Source: CAD feature listing. Evaluate the final solid. Frame: model axes, mm. Face numbers are marked on the shaded views. A direction names the side the tool comes from. Round coordinates to 2 decimals unless told otherwise and drop trailing zeros. Order: outer loops, then holes, each group sorted by start corner. A loop starts at its lowest first (then second) coordinate and runs counter-clockwise, first axis right, second up. Notation, with made-up numbers: (-26.5, 33.25) - (15.5, 33.25) arc R17 cw to (15.5, 37.25) - close; hole circle Ø8 at (-5, 14.5). An arc over 180 degrees is marked (long way). Put each result on its own line as item: value. Start each with the question number.
1) Access query for the marked faces 4 and 5. Directions: +Z, -Z, +X, -X, +Y, -Y. A direction counts if a zero-diameter tool reaches every point of the face in a straight line with its end or side. Return the directions, or none.
2) Section A-A on x = 5. Output: boundary loops of the cut face in (y, z).
3) Line query: probe 1 along X at (y, z) = (-2.5, 4); probe 2 along Z at (x, y) = (5, -8); probe 3 along X at (y, z) = (10.75, 5.25). Output: solid intervals per line, ascending. Write a range as [from, to].
4) Contact query for a flat-ended pin moving along its axis: P1, Ø4.5, axis at x = -5, z = 4, coming from the +Y side. Output: stop coordinate, or through.
5) Section B-B on y = -9. Output: boundary loops of the cut face in (x, z).
6) Mould query, pull axis X, two halves, no side actions, for the marked faces 1, 2 and 3. Classes: +X half, -X half, draft (parallel to the pull), parting line (faces both ways), or undercut.
7) Section C-C on z = 3.5. State how many separate pieces and enclosed holes the cut face has, then the cut area to 3 significant figures.
8) Section D-D on x = 12. Output: boundary loops of the cut face in (y, z) (3 decimals).
```python
from build123d import *

# Parameters (mm, degrees)
BOSS_EXTRU_1_DEPTH      = 8
ENL_V_MAT_EXTRU_1_REACH = 27
ESQUISSE2_R             = 2
CHANFREIN1_SIZE         = 1
CONG_1_R                = 2


with BuildPart() as part:
    # Esquisse1 → Boss.-Extru.1 (new body)
    with BuildSketch(Plane.XY):
        with BuildLine():
            Line((-17, 12.5), (-17, -4.5))
            ThreePointArc((-17, -4.5), (-11.343145751, -6.843145751), (-9, -12.5))
            Line((-9, -12.5), (9, -12.5))
            ThreePointArc((9, -12.5), (11.343145751, -6.843145751), (17, -4.5))
            Line((17, -4.5), (17, 12.5))
            Line((17, 12.5), (13.4, 12.5))
            ThreePointArc((13.4, 12.5), (0, -0.9), (-13.4, 12.5))
            Line((-13.4, 12.5), (-17, 12.5))
        make_face()
    extrude(amount=BOSS_EXTRU_1_DEPTH)

    # Esquisse2 → Enlèv. mat.-Extru.1 (cut, up to next)
    with BuildSketch(Plane.XZ.offset(12.5), mode=Mode.PRIVATE) as enl_v_mat_extru_1_sk1:
        with Locations((-5, 4)):
            Circle(ESQUISSE2_R)
    enl_v_mat_extru_1_tool1 = extrude(enl_v_mat_extru_1_sk1.sketch, amount=-ENL_V_MAT_EXTRU_1_REACH, mode=Mode.PRIVATE) & part.part
    add(enl_v_mat_extru_1_tool1.solids().sort_by_distance((-5, -12.5, 4))[0], mode=Mode.SUBTRACT)
    # Esquisse2 → Enlèv. mat.-Extru.1 (cut, up to next)
    with BuildSketch(Plane.XZ.offset(12.5), mode=Mode.PRIVATE) as enl_v_mat_extru_1_sk2:
        with Locations((5, 4)):
            Circle(ESQUISSE2_R)
    enl_v_mat_extru_1_tool2 = extrude(enl_v_mat_extru_1_sk2.sketch, amount=-ENL_V_MAT_EXTRU_1_REACH, mode=Mode.PRIVATE) & part.part
    add(enl_v_mat_extru_1_tool2.solids().sort_by_distance((5, -12.5, 4))[0], mode=Mode.SUBTRACT)

    # Chanfrein1
    chanfrein1_edges = [part.edges().sort_by_distance(p)[0] for p in [
        (-7, -12.5, 4),
        (3, -12.5, 4),
    ]]
    chamfer(chanfrein1_edges, length=CHANFREIN1_SIZE)

    # Congé1
    cong_1_edges = [part.edges().sort_by_distance(p)[0] for p in [
        (-13.4, 12.5, 4),
        (13.4, 12.5, 4),
    ]]
    fillet(cong_1_edges, radius=CONG_1_R)


solid = part.part
```
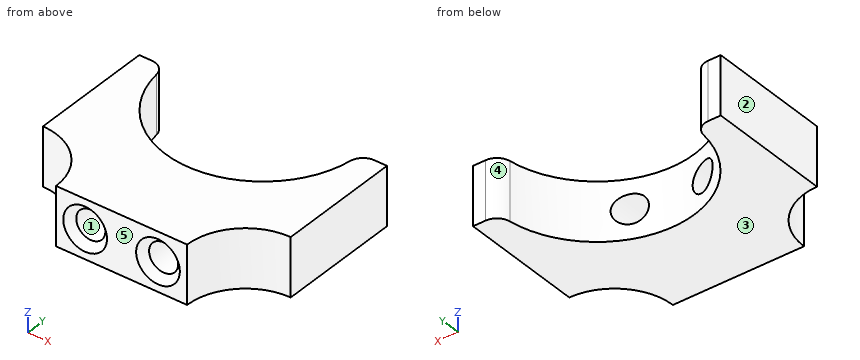
Answer sheet:
1. face 4: +Z, -Z, +Y
1. face 5: +Z, -Z, +X, -X, -Y
2. outline: (-12.5, 0) - (0.07, 0) - (0.07, 2) - (-11.5, 2) - (-12.5, 1) - close; (-12.5, 7) - (-11.5, 6) - (0.07, 6) - (0.07, 8) - (-12.5, 8) - close
3. probe 1: [-17, -7], [-3, 3], [7, 17]
3. probe 2: [0, 2], [6, 8]
3. probe 3: [-17, -13.29], [13.29, 17]
4. P1: y = 1.23
5. outline: (-9.81, 0) - (9.81, 0) - (9.81, 8) - (-9.81, 8) - close; hole circle Ø4 at (-5, 4); hole circle Ø4 at (5, 4)
6. face 1: undercut
6. face 2: -X half
6. face 3: draft
7. separate pieces: 3
7. enclosed holes: 0
7. area: 366 mm^2
8. outline: (-6.255, 0) - (6.537, 0) - (6.537, 8) - (-6.255, 8) - close
